from build123d import *

# Parameters (mm, degrees)
F0_W     = 14.33
F0_H     = 14.33
F0_W_2   = 10.33
F0_H_2   = 10.33
F0_W_3   = 6.33
F0_H_3   = 6.33
F1_DEPTH = 2
F2_W     = 10.33
F2_H     = 10.33
F3_DEPTH = 14
F4_R     = 3
F5_DEPTH = 2
F6_W     = 0.835
F6_H     = 12
F6_W_2   = 10.33
F7_DEPTH = 6


with BuildPart() as f1:
    # F0 (on Top) → F1 (new body)
    with BuildSketch(Plane.XY):
        with Locations((-14.33, 0)):
            Rectangle(F0_W, F0_H)
        with Locations((-14.33, 0)):
            Rectangle(F0_W_2, F0_H_2, mode=Mode.SUBTRACT)
        Rectangle(F0_W, F0_H)
        Rectangle(F0_W_2, F0_H_2, mode=Mode.SUBTRACT)
        Rectangle(F0_W_2, F0_H_2)
        Rectangle(F0_W_3, F0_H_3, mode=Mode.SUBTRACT)
        Rectangle(F0_W_3, F0_H_3)
        with Locations((14.33, 0)):
            Rectangle(F0_W, F0_H)
        with Locations((14.33, 0)):
            Rectangle(F0_W_2, F0_H_2, mode=Mode.SUBTRACT)
    extrude(amount=F1_DEPTH)

    # F2 (on face) → F3 (join)
    with BuildSketch(Plane.XY.offset(2)):
        Polygon((-7.165, 7.165), (-21.495, 7.165), (-21.495, -7.165), (-7.165, -7.165), (7.165, -7.165), (21.495, -7.165), (21.495, 7.165), (7.165, 7.165), align=None)
        with Locations((-14.33, 0)):
            Rectangle(F2_W, F2_H, mode=Mode.SUBTRACT)
        Rectangle(F2_W, F2_H, mode=Mode.SUBTRACT)
        with Locations((14.33, 0)):
            Rectangle(F2_W, F2_H, mode=Mode.SUBTRACT)
    extrude(amount=F3_DEPTH)

    # F4 (on face) → F5 (join)
    with BuildSketch(Plane.XY.offset(16)):
        Polygon((21.495, 7.165), (7.165, 7.165), (-7.165, 7.165), (-21.495, 7.165), (-21.495, -7.165), (-7.165, -7.165), (7.165, -7.165), (21.495, -7.165), align=None)
        with Locations((-14.33, 0)):
            Circle(F4_R, mode=Mode.SUBTRACT)
        with Locations((14.33, 0)):
            Circle(F4_R, mode=Mode.SUBTRACT)
    extrude(amount=F5_DEPTH)

    # F6 (on face) → F7 (cut)
    with BuildSketch(Plane.YZ.offset(9.165)):
        with Locations((-5.5825, 9)):
            Rectangle(F6_W, F6_H)
        with Locations((0, 9)):
            Rectangle(F6_W_2, F6_H)
        with Locations((5.5825, 9)):
            Rectangle(F6_W, F6_H)
    extrude(amount=-F7_DEPTH, mode=Mode.SUBTRACT)


solid = f1.part
Source: CAD feature listing. Evaluate the final solid. Frame: model axes, mm. A direction names the side the tool comes from. Coordinates: 2 decimals unless noted, no trailing zeros. Order: outer loops, then holes, each group sorted by start corner. A loop starts at its lowest first (then second) coordinate and runs counter-clockwise, first axis right, second up. Notation, with made-up numbers: M 1,24.25 L 44,24.25 A20 ccw 44,57.25 Z; hole C -29,66.5 d8. An arc over 180 degrees is marked long. Write each question's results on one line, items separated by ' | '. Start each with the question number.
Item 1: Cut plane B-B (z = 8.25). Return loops of the section in (x, y) (3 decimals), and give its area (3 significant figures).
Item 2: Line query: probe 1 along Y at (x, z) = (14.33, 17.25) (3 decimals); probe 2 along X at (y, z) = (-1, 16.25) (3 decimals); probe 3 along Z at (x, y) = (8, -4). Output: solid intervals per line, ascending.
Item 3: Cut plane C-C (x = 14.33). Return loops of the section in (y, z) (3 decimals), and give its area (3 significant figures).
Item 4: Cut plane A-A (y = 0). Return loops of the section in (x, z) (3 decimals).
Item 5: Cut plane D-D (y = -4.5). Return loops of the section in (x, z) (3 decimals).
Item 6: First-contact query: pin 1 Ø8 at (x, y) = (14, -1.5) entering from -Z; pin 2 Ø7 at (x, y) = (-14.33, 0) entering from -Z. Flat tips, straight axial feed; report the tip coordinate or a pass-through.
Item 7: Set-up query: faces 1 (the face through (14, -5.165, 8)), 2 (the face through (0, 0, 16)), 3 (the face through (21.495, 0, 9)). Return all of +Z, -Z, +X, -X, +Y, -Y with unobstructed straight access to the full face (end or side cutting, diameter ignored); none if empty.
Item 8: Draft query along Y for faces 4 (the face through (0, -7.165, 9)), 5 (the face through (0, 7.165, 9)), 6 (the face through (0, 0, 2)). Return one class per face: pulls with the +Y half, pulls with the -Y half, needs draft (parallel to the pull), parting line crosses it, or undercut.
Checked values:
1) outline: M -21.495,-7.165 L 21.495,-7.165 L 21.495,7.165 L -21.495,7.165 Z; hole M -19.495,-5.165 L -9.165,-5.165 L -9.165,5.165 L -19.495,5.165 Z; hole M -5.165,-5.165 L 3.165,-5.165 L 3.165,-6 L 9.165,-6 L 9.165,-5.165 L 19.495,-5.165 L 19.495,5.165 L 9.165,5.165 L 9.165,6 L 3.165,6 L 3.165,5.165 L -5.165,5.165 Z | area: 245 mm2
2) probe 1: y = -7.165 to -3, 3 to 7.165 | probe 2: x = -21.495 to -17.158, -11.502 to 11.502, 17.158 to 21.495 | probe 3: z = 0 to 3, 15 to 18
3) outline: M -7.165,0 L -5.165,0 L -5.165,16 L -3,16 L -3,18 L -7.165,18 Z; M 3,16 L 5.165,16 L 5.165,0 L 7.165,0 L 7.165,18 L 3,18 Z | area: 80.7 mm2
4) outline: M -21.495,0 L -19.495,0 L -19.495,16 L -17.33,16 L -17.33,18 L -21.495,18 Z; M -11.33,16 L -9.165,16 L -9.165,0 L 9.165,0 L 9.165,3 L 5.165,3 L 5.165,2 L -5.165,2 L -5.165,16 L 5.165,16 L 5.165,15 L 9.165,15 L 9.165,16 L 11.33,16 L 11.33,18 L -11.33,18 Z; M 17.33,16 L 19.495,16 L 19.495,0 L 21.495,0 L 21.495,18 L 17.33,18 Z
5) outline: M -21.495,0 L -19.495,0 L -19.495,16 L -9.165,16 L -9.165,0 L 9.165,0 L 9.165,3 L 5.165,3 L 5.165,2 L -5.165,2 L -5.165,16 L 5.165,16 L 5.165,15 L 9.165,15 L 9.165,16 L 19.495,16 L 19.495,0 L 21.495,0 L 21.495,18 L -21.495,18 Z
6) pin 1: stops at z = 0 | pin 2: stops at z = 16
7) face 1: -Z | face 2: none | face 3: +Z, -Z, +X, +Y, -Y
8) face 4: pulls with the -Y half | face 5: pulls with the +Y half | face 6: undercut
